Could you check a few things on this model? Use its own coordinates, in mm. Face numbers are marked on the shaded views. Give positions to 0.01 mm unless a question says otherwise; leave off trailing zeros. Write each loop counter-clockwise with the first axis right and the second up, starting at its lowest first coordinate (ties: lowest second). Pieces come first, ordered by that corner, then holes. Notation, with made-up numbers: M -22,-37 L 18,-37 A9 ccw 18,-30 Z; hole C -39,26 d2. An arc over 180 degrees is marked long. Answer as a JSON object with one key per item and string values. Group by question number.
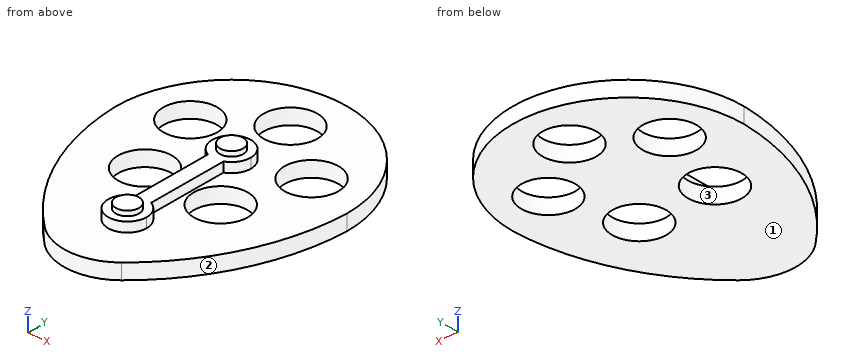
```python
from build123d import *

# Parameters (mm, degrees)
F0_R     = 8.89
F1_DEPTH = 5.08
F3_R     = 19.05
F4_DEPTH = 3.175
F5_R     = 3.81
F6_DEPTH = 1.6002


with BuildPart() as f1:
    # F0 (on Top) → F1 (new body)
    with BuildSketch(Plane.XY):
        with BuildLine():
            ThreePointArc((0, -63.5), (27.2824792884, -36.689487573), (38.1, 0))
            ThreePointArc((38.1, 0), (0, 38.1), (-38.1, 0))
            ThreePointArc((-38.1, 0), (-27.2824792884, -36.689487573), (0, -63.5))
        make_face()
        with Locations((-13.1279943906, -17.1087353843)):
            Circle(F0_R, mode=Mode.SUBTRACT)
        with Locations((12.3692268928, -17.6650867319)):
            Circle(F0_R, mode=Mode.SUBTRACT)
        with Locations((-20.264554991, 7.3756948274)):
            Circle(F0_R, mode=Mode.SUBTRACT)
        with Locations((0, 21.5650889905)):
            Circle(F0_R, mode=Mode.SUBTRACT)
        with Locations((20.5669909147, 6.4847473263)):
            Circle(F0_R, mode=Mode.SUBTRACT)
    extrude(amount=F1_DEPTH)

    # F3
    f3_edges = [f1.edges().sort_by_distance(p)[0] for p in [
        (0, -63.5, 2.54),
    ]]
    fillet(f3_edges, radius=F3_R)

    # F2 (on face) → F4 (join)
    with BuildSketch(Plane.XY.offset(5.08)):
        with BuildLine():
            ThreePointArc((2.4886815787, -5.842), (5.2974346633, -3.5013834391), (6.35, 0))
            ThreePointArc((6.35, 0), (-3.5013834391, 5.2974346633), (-2.4886815787, -5.842))
            ThreePointArc((-2.4886815787, -5.842), (0, -6.35), (2.4886815787, -5.842))
        make_face()
        with BuildLine():
            ThreePointArc((2.4886815787, -5.842), (0, -6.35), (-2.4886815787, -5.842))
            Line((-2.4886815787, -5.842), (-2.4886815787, -32.258))
            ThreePointArc((-2.4886815787, -32.258), (-1.27, -31.8782960533), (0, -31.75))
            ThreePointArc((0, -31.75), (1.3248127312, -31.8897366218), (2.5913184213, -32.3027964639))
            Line((2.5913184213, -32.3027964639), (2.5913184213, -5.842))
            Line((2.5913184213, -5.842), (2.4886815787, -5.842))
        make_face()
        with BuildLine():
            ThreePointArc((0, -31.75), (-1.27, -31.8782960533), (-2.4886815787, -32.258))
            ThreePointArc((-2.4886815787, -32.258), (-3.5013834391, -43.3974346633), (6.35, -38.1))
            ThreePointArc((6.35, -38.1), (5.3281034138, -34.6454647183), (2.5913184213, -32.3027964639))
            Line((2.5913184213, -32.3027964639), (0, -31.75))
        make_face()
        with BuildLine():
            ThreePointArc((2.5913184213, -32.3027964639), (1.3248127312, -31.8897366218), (0, -31.75))
            Line((0, -31.75), (2.5913184213, -32.3027964639))
        make_face()
    extrude(amount=F4_DEPTH)

    # F5 (on face) → F6 (join)
    with BuildSketch(Plane.XY.offset(8.255)):
        with Locations((0, -38.1)):
            Circle(F5_R)
        Circle(F5_R)
    extrude(amount=F6_DEPTH)


solid = f1.part
```
1) If we section it at B-B, the plane z = 7: List the corners of the cut face in (x, y) for me, plus the area to 3 significant figures.
2) If we section it at C-C, the plane y = 28.5: List the corners of the cut face in (x, z) for me, plus the area to 3 significant figures.
3) I'm going to push flat-ended pins straight in: pin 1 (14 mm diameter, centred on x = -3, y = -17, fed in from +Z) (3 decimals); pin 2 (1 mm diameter, centred on y = -14.5, z = 7, fed in from +X); pin 3 (5 mm diameter, centred on y = -36, z = 5.5, fed in from -X). Where does each tip first touch, or does it pass through?
4) We'd pull the mould along Y, two halves only. Please class the marked faces 1, 2 and 3: released by +Y, released by -Y, zero draft, split by the parting line, or undercut.
5) If we section it at A-A, the plane x = -24: List the corners of the cut face in (y, z) for me, plus the area to 3 significant figures.
6) Please list where these lines run through material, in increasing order: line 1 along Y through (x, z) = (0, 1.4); line 2 along Y through (x, z) = (-5.5, 1.25); line 3 along X through (y, z) = (-23, 3.75). Write a range as from..to.
7) If we section it at D-D, the plane z = 2: Give the number of separate pieces and of enclosed holes in the cut face, plus the area to 3 significant figures.
Taken from the geometry:
{
 "1": {"outline": "M -2.49,-32.26 A6.35 ccw long 2.59,-32.3 L 2.59,-5.84 L 2.49,-5.84 A6.35 ccw long -2.49,-5.84 Z", "area": "384 mm²"},
 "2": {"outline": "M -25.29,0 L -5.56,0 L -5.56,5.08 L -25.29,5.08 Z; M 5.56,0 L 25.29,0 L 25.29,5.08 L 5.56,5.08 Z", "area": "200 mm²"},
 "3": {"pin 1": "z = 8.255", "pin 2": "x = 2.59", "pin 3": "x = -29.07"},
 "4": {"face 1": "zero draft", "face 2": "released by -Y", "face 3": "undercut"},
 "5": {"outline": "M -41.7,0 L -0.69,0 L -0.69,5.08 L -41.7,5.08 Z; M 15.44,0 L 29.59,0 L 29.59,5.08 L 15.44,5.08 Z", "area": "280 mm²"},
 "6": {"line 1": "-59.17..12.68, 30.46..38.1", "line 2": "-58.36..-21.67, -12.54..14.58, 28.55..37.7", "line 3": "-33.74..-19.79, -6.47..5.26, 19.48..33.74"},
 "7": {"separate pieces": "1", "enclosed holes": "5", "area": "4,380 mm²"}
}
